from build123d import *

# Parameters (mm, degrees)
ESQUISSE3_R             = 7
BOSS_EXTRU_2_DEPTH      = 5
BOSS_EXTRU_3_DEPTH      = 45
ENL_V_START             = -73.880031702
ENL_V_MAT_EXTRU_3_DEPTH = 78.880031702
ESQUISSE4_4_W           = 16.307493561
ESQUISSE4_4_H           = 0.792049354
ENL_V_MAT_EXTRU_4_DEPTH = 58.619847767
ENL_V_MAT_EXTRU_6_DEPTH = 57.248456757
ENL_V_MAT_EXTRU_7_DEPTH = 58.619847767


with BuildPart() as part:
    # Esquisse3 → Boss.-Extru.2 (new body)
    with BuildSketch(Plane.XY):
        Circle(ESQUISSE3_R)
    extrude(amount=BOSS_EXTRU_2_DEPTH)

    # Esquisse3_3 → Boss.-Extru.3 (add)
    with BuildSketch(Plane.XY):
        with BuildLine():
            ThreePointArc((-6.556240583, 2.452694319), (-31.795381091, -9.503990443), (-43.059714875, -35.059641647))
            Line((-43.059714875, -35.059641647), (-29.67043681, -37.846531887))
            Line((-29.67043681, -37.846531887), (-28.42882324, -31.881349224))
            Line((-28.42882324, -31.881349224), (-37.880972605, -29.913946449))
            ThreePointArc((-37.880972605, -29.913946449), (-26.825365644, -10.900303142), (-6.699170831, -2.030051767))
            ThreePointArc((-6.699170831, -2.030051767), (-6.99644453, 0.22307834), (-6.556240583, 2.452694319))
        make_face()
    boss_extru_3 = extrude(amount=BOSS_EXTRU_3_DEPTH)

    # Esquisse4 → Enl_v. mat.-Extru.3 (cut)
    with BuildSketch(Plane(origin=(0, 0, 0), x_dir=(1, 0, 0), z_dir=(0, 1, 0)).offset(ENL_V_START)):
        Polygon((-6.556240583, -21.643777245), (-6.556240583, -5), (-22.534905521, -5), (-22.534905521, -5.792049354), (-43.059714875, -5.792049354), (-43.059714875, -11.918484986), (-43.059714875, -45), (-43.059714875, -53.527020644), (-6.425184121, -53.527020644), align=None)
    enl_v_mat_extru_3 = extrude(amount=ENL_V_MAT_EXTRU_3_DEPTH, mode=Mode.SUBTRACT)

    # Esquisse4_4 → Enl_v. mat.-Extru.4 (cut, through all)
    with BuildSketch(Plane(origin=(0, 0, 0), x_dir=(1, 0, 0), z_dir=(0, 1, 0))):
        with Locations((-34.905968095, -0.396024677)):
            Rectangle(ESQUISSE4_4_W, ESQUISSE4_4_H)
    enl_v_mat_extru_4 = extrude(amount=-ENL_V_MAT_EXTRU_4_DEPTH, mode=Mode.SUBTRACT)

    # Esquisse5 → Enl_v. mat.-Extru.6 (cut, through all)
    with BuildSketch(Plane(origin=(-7.540837864, -36.229046112, 0), x_dir=(0.9790175257089632, -0.2037760642340011, 0), z_dir=(0.2037760642340011, 0.9790175257089632, 0))):
        with BuildLine():
            Line((-25.202181908, -0.792049354), (-21.33566032, -0.792049354))
            Line((-21.33566032, -0.792049354), (-21.33566032, -5.792049354))
            ThreePointArc((-21.33566032, -5.792049354), (-22.966477925, -3.05816873), (-25.202181908, -0.792049354))
        make_face()
    enl_v_mat_extru_6 = extrude(amount=-ENL_V_MAT_EXTRU_6_DEPTH, mode=Mode.SUBTRACT)

    # Sym_trie1: Boss.-Extru.3, Enl_v. mat.-Extru.3, Enl_v. mat.-Extru.4, Enl_v. mat.-Extru.6 across plane
    add(boss_extru_3.mirror(Plane.XY.offset(2.5)))
    add(enl_v_mat_extru_3.mirror(Plane.XY.offset(2.5)), mode=Mode.SUBTRACT)
    add(enl_v_mat_extru_4.mirror(Plane.XY.offset(2.5)), mode=Mode.SUBTRACT)
    add(enl_v_mat_extru_6.mirror(Plane.XY.offset(2.5)), mode=Mode.SUBTRACT)

    # Esquisse6 → Enl_v. mat.-Extru.7 (cut, through all)
    with BuildSketch(Plane(origin=(0, 0, 0), x_dir=(1, 0, 0), z_dir=(0, 1, 0))):
        Polygon((-22.534905521, -1196.824915859), (-22.534905521, -5), (-43.059714875, -5), (-43.059714875, -5.792049354), (-28.70402214, -5.792049354), align=None)
    extrude(amount=-ENL_V_MAT_EXTRU_7_DEPTH, mode=Mode.SUBTRACT)


solid = part.part
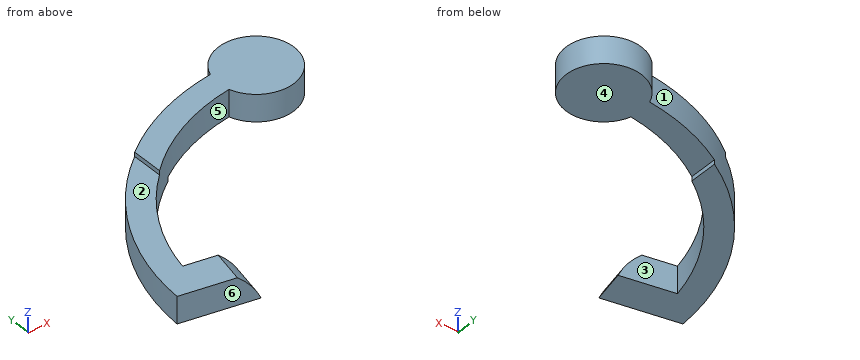
The listing builds one solid part. Answer for the finished solid, in the listing's coordinates (mm). Face numbers are marked on the shaded views. A direction names the side the tool comes from. Coordinates: 2 decimals unless noted, no trailing zeros. Loops run counter-clockwise (first coordinate to the right, second up) from the corner with the lowest first, then second, coordinate; pieces in that order, holes last. Notation, with made-up numbers: (68.5, 55.25) -> (86.5, 55.25) arc R15 cw to (86.5, 69.25) -> close; hole circle Ø4 at (-22.5, 11.5). An arc over 180 degrees is marked (long way). Answer in a Markdown table with one row per item. Add a question column.
1. Determine the mould class of the marked faces 4, 5 and 6 for opening direction Y: +Y half, -Y half, draft (parallel to the pull), parting line (faces both ways), or undercut.
2. The part is cut by section B-B, the plane x = 0. Write down the section's boundary in (y, z).
3. The part is cut by section C-C, the plane z = 2.2. Write down the section's boundary in (x, y), then the cut area to 3 significant figures.
4. For the marked faces 1, 2 and 3, determine the directions among +Z, -Z, +X, -X, +Y, -Y from which every point of the face is accessible in a straight line to the end or side of a thin tool.
5. Consider line 1 (Z direction, x = -34, y = -34); line 2 (X direction, y = -5.5, z = 3.05); line 3 (X direction, y = -6, z = 2.6). Determine where each line is inside the solid, lowest interval first. Write a range as [from, to].
6. The part is cut by section D-D, the plane y = -22. Write down the section's boundary in (x, z).
7. The part is cut by section A-A, the plane y = -4. Write down the section's boundary in (x, z).
8. Flat-ended cylindrical pins translate along their axes: P1, Ø1, axis at y = -16, z = 1, coming from the +X side; P2, Ø0.9, axis at y = -5.5, z = -0.5, coming from the +X side; P3, Ø5, axis at x = -32, y = -23, coming from the +Z side; P4, Ø1, axis at x = -29, z = 2, coming from the +Y side. Find the tip coordinate at first contact, or state that the pin passes through.
Answer below:
| question | item | result |
|---|---|---|
| 1 | face 4 | draft |
| 1 | face 5 | undercut |
| 1 | face 6 | -Y half |
| 2 | outline | (-7, 0) -> (7, 0) -> (7, 5) -> (-7, 5) -> close |
| 3 | outline | (-43.06, -35.06) -> (-31.47, -37.47) -> (-30.23, -31.51) -> (-37.88, -29.91) arc R35.55 cw to (-6.7, -2.03) arc R7 ccw (long way) to (-6.56, 2.45) arc R40 ccw to start |
| 3 | area | 440 mm2 |
| 4 | face 1 | +Z, -Z, -X, +Y |
| 4 | face 2 | +Z, -X, +Y, -Y |
| 4 | face 3 | +Z, -Z, +X |
| 5 | line 1 | [-0.79, 4.21] |
| 5 | line 2 | [-27.26, -18.82], [-4.33, 4.33] |
| 5 | line 3 | [-27.91, -19.8], [-3.61, 3.61] |
| 6 | outline | (-40.04, -0.79) -> (-35.17, -0.79) -> (-35.17, 4.21) -> (-40.04, 4.21) -> close |
| 7 | outline | (-25.14, -0.79) -> (-22.53, -0.79) -> (-22.53, 0) -> (-15.3, 0) -> (-15.3, 5) -> (-25.14, 5) -> close; (-5.74, 0) -> (5.74, 0) -> (5.74, 5) -> (-5.74, 5) -> close |
| 8 | P1 | x = -31.13 |
| 8 | P2 | x = -22.53 |
| 8 | P3 | through |
| 8 | P4 | y = -6.48 |
